```python
from build123d import *

# Parameters (mm, degrees)
SKETCH_W     = 20.4
SKETCH_H     = 37.336792
PAD_DEPTH    = 7
SKETCH001_W  = 8
SKETCH001_H  = 8
POCKET_DEPTH = 7
CHAMFER_SIZE = 2


with BuildPart() as part:
    # Sketch → Pad (new body)
    with BuildSketch(Plane.XY):
        Rectangle(SKETCH_W, SKETCH_H)
        Polygon((3.85, 3.331604), (7.7, 10), (3.85, 16.668396), (-3.85, 16.668396), (-7.7, 10), (-3.85, 3.331604), align=None, mode=Mode.SUBTRACT)
        Polygon((3.85, -3.331604), (-3.85, -3.331604), (-7.7, -10), (-3.85, -16.668396), (3.85, -16.668396), (7.7, -10), align=None, mode=Mode.SUBTRACT)
    extrude(amount=PAD_DEPTH)

    # Sketch001 → Pocket (cut)
    with BuildSketch(Plane.XY.offset(7)):
        with Locations((7.7, 10)):
            Rectangle(SKETCH001_W, SKETCH001_H)
    pocket = extrude(amount=-POCKET_DEPTH, mode=Mode.SUBTRACT)

    # Mirrored: Pocket across Sketch001 H_Axis
    add(pocket.mirror(Plane(origin=(0, 0, 7), x_dir=(0, 0, 1), z_dir=(0, 1, 0))), mode=Mode.SUBTRACT)

    # Chamfer
    chamfer_edges = [part.edges().sort_by_distance(p)[0] for p in [
        (-10.2, 18.668396, 3.5),
        (10.2, 18.668396, 3.5),
        (-10.2, -18.668396, 3.5),
        (10.2, 14, 3.5),
        (10.2, -18.668396, 3.5),
        (10.2, 6, 3.5),
        (10.2, -6, 3.5),
        (10.2, -14, 3.5),
    ]]
    chamfer(chamfer_edges, length=CHAMFER_SIZE)


solid = part.part
```
Could you check a few things on this model? Use its own coordinates, in mm. A direction names the side the tool comes from. Give positions to 0.01 mm unless a question says otherwise; leave off trailing zeros. Order: outer loops, then holes, each group sorted by start corner. A loop starts at its lowest first (then second) coordinate and runs counter-clockwise, first axis right, second up.
Q1. Suppose I cut it at C-C, the plane y = -14.5. Write out the boundary of the cut face in (x, z), and give its area (3 significant figures).
Q2. For faces 4 (the flat face through (-5.8, -13.29, 3.45)), 5 (the flat face through (9.2, -5, 3.5)), 6 (the flat face through (9.214, 17.654, 3.451)), which set-ups out of +Z, -Z, +X, -X, +Y, -Y let a thin tool reach every point of the face, with its end or its side?
Q3. We'd pull the mould along X, two halves only. Please class faces 1 (the flat face through (0, 18.668, 3)), 2 (the flat face through (10.2, 0, 3)), 3 (the flat face through (4.61, -15.35, 3.45)): +X half, -X half, draft (parallel to the pull), parting line (faces both ways), or undercut.
Q4. I'm going to push a flat-ended pin straight in: P1, Ø2, axis at x = -4, y = -5, coming from the +Z side. Where does the tip first touch, or does it pass through?
Q5. Suppose I cut it at A-A, the plane x = -0.5. Write out the boundary of the cut face in (y, z), and give its area (3 significant figures).
Q6. If I drill on line 1 along Y through (x, z) = (-1, 0.75); line 2 along Y through (x, z) = (7.75, 4.75); line 3 along X through (y, z) = (16.5, 3.75), over which ranges is the centre line in solid material (lowest first)?
Q7. Suppose I cut it at D-D, the plane x = 4.5. Write out the boundary of the cut face in (y, z).
Solution:
1. outline: (-10.2, 0) - (-5.1, 0) - (-5.1, 7) - (-10.2, 7) - close; (5.1, 0) - (8.7, 0) - (8.7, 7) - (5.1, 7) - close
1. area: 60.9 mm2
2. face 4: +Z, -Z
2. face 5: +Z, -Z, +X
2. face 6: +Z, -Z, +X, +Y
3. face 1: draft
3. face 2: +X half
3. face 3: undercut
4. P1: stops at z = 7
5. outline: (-18.67, 0) - (-16.67, 0) - (-16.67, 7) - (-18.67, 7) - close; (-3.33, 0) - (3.33, 0) - (3.33, 7) - (-3.33, 7) - close; (16.67, 0) - (18.67, 0) - (18.67, 7) - (16.67, 7) - close
5. area: 74.6 mm2
6. line 1: y = -18.67 to -16.67, -3.33 to 3.33, 16.67 to 18.67
6. line 2: y = -18.67 to -14, -6 to 6, 14 to 18.67
6. line 3: x = -10.2 to -3.95, 3.95 to 10.2
7. outline: (-18.67, 0) - (-15.54, 0) - (-15.54, 7) - (-18.67, 7) - close; (-4.46, 0) - (4.46, 0) - (4.46, 7) - (-4.46, 7) - close; (15.54, 0) - (18.67, 0) - (18.67, 7) - (15.54, 7) - close
